Input: part model. Units: mm. Frame: model coordinates. A direction names the side the tool comes from. Give positions to 0.01 mm unless a question says otherwise; leave off trailing zeros. Write each loop counter-clockwise with the first axis right and the second up, starting at its lowest first coordinate (ties: lowest second). Pieces come first, ordered by that corner, then holes. Notation, with made-up numbers: (47.5, -37) - (105.5, -37) arc R35 ccw to (105.5, -3) - close; hole circle Ø6 at (-38, 36). An arc over 180 degrees is marked (long way). Use a Markdown table: item, result. Add a question column.
1. Section query A-A, the plane y = 0. Return loops of the section in (x, z), plus the area to 3 significant figures.
2. Section query C-C, the plane z = -1.5. Return loops of the section in (x, y), plus the area to 3 significant figures.
3. Set-up query: faces 1 (the flat face through (-0.1, -12.4, -3)), 2 (the flat face through (-5.3, 15.3, 4)). Return all of +Z, -Z, +X, -X, +Y, -Y with unobstructed straight access to the full face (end or side cutting, diameter ignored); none if empty.
4. Material intervals for probe 1 along Y at (x, z) = (0, -1); probe 2 along Z at (x, y) = (-1.5, -1); probe 3 along Z at (x, y) = (-10, -10), sorted ascending.
5. Pin query (flat end, axial travel): pin 1 (10 mm diameter, centred on x = -18, y = -15.5, fed in from -Z); pin 2 (1 mm diameter, centred on x = 6.5, z = 10, fed in from -Y); pin 3 (1.5 mm diameter, centred on y = -18, z = 12, fed in from +X). Return the tip coordinate at first contact, or that it passes through.
6. Mould query, pull axis Y, two halves, no side actions, for faces 3 (the flat face through (1.11, -14.11, 3)), 4 (the flat face through (0, 0, 4)), 5 (the cylindrical face through (10.382, -19.961, 8.93)). Classes: released by +Y, released by -Y, zero draft, split by the parting line, or undercut.
7. Section query D-D, the plane x = 18. Return loops of the section in (y, z), plus the area to 3 significant figures.
```python
from build123d import *

# Parameters (mm, degrees)
SKETCH_1_R      = 14
SKETCH_1_R_2    = 12.25
EXTRUDE_1_DEPTH = 3
SKETCH_2_R      = 15.963029432
SKETCH_2_R_2    = 12.25
EXTRUDE_2_DEPTH = 1
SKETCH_3_R      = 22.5
EXTRUDE_3_DEPTH = 10


with BuildPart() as part:
    # 草图1 → 凸台-拉伸1 (new, symmetric)
    with BuildSketch(Plane.XY):
        Circle(SKETCH_1_R)
        Circle(SKETCH_1_R_2, mode=Mode.SUBTRACT)
    extrude(amount=EXTRUDE_1_DEPTH, both=True)

    # 草图2 → 凸台-拉伸2 (add)
    with BuildSketch(Plane.XY.offset(3)):
        Circle(SKETCH_2_R)
        Circle(SKETCH_2_R_2, mode=Mode.SUBTRACT)
    extrude(amount=EXTRUDE_2_DEPTH)

    # 草图3 → 凸台-拉伸3 (add)
    with BuildSketch(Plane.XY.offset(4)):
        Circle(SKETCH_3_R)
    extrude(amount=EXTRUDE_3_DEPTH)


solid = part.part
```
Result sheet:
| question | item | result |
|---|---|---|
| 1 | outline | (-22.5, 4) - (-15.96, 4) - (-15.96, 3) - (-14, 3) - (-14, -3) - (-12.25, -3) - (-12.25, 4) - (12.25, 4) - (12.25, -3) - (14, -3) - (14, 3) - (15.96, 3) - (15.96, 4) - (22.5, 4) - (22.5, 14) - (-22.5, 14) - close |
| 1 | area | 478 mm² |
| 2 | outline | circle Ø28 at (0, 0); hole circle Ø24.5 at (0, 0) |
| 2 | area | 144 mm² |
| 3 | face 1 | -Z, +X, -X, +Y, -Y |
| 3 | face 2 | -Z |
| 4 | probe 1 | y = -14 to -12.25, 12.25 to 14 |
| 4 | probe 2 | z = 4 to 14 |
| 4 | probe 3 | z = 3 to 14 |
| 5 | pin 1 | stops at z = 4 |
| 5 | pin 2 | stops at y = -21.69 |
| 5 | pin 3 | stops at x = 14.45 |
| 6 | face 3 | zero draft |
| 6 | face 4 | undercut |
| 6 | face 5 | split by the parting line |
| 7 | outline | (-13.5, 4) - (13.5, 4) - (13.5, 14) - (-13.5, 14) - close |
| 7 | area | 270 mm² |
